Input: part model. Units: mm. Frame: model coordinates. A direction names the side the tool comes from. Coordinates: 2 decimals unless noted, no trailing zeros. Order: outer loops, then holes, each group sorted by start corner. A loop starts at its lowest first (then second) coordinate and runs counter-clockwise, first axis right, second up. Notation, with made-up numbers: (75, 54.5) - (112, 54.5) arc R8 cw to (112, 67.5) - close; hole circle Ø10 at (-7.5, -18). An arc over 180 degrees is marked (long way). Answer as CSV lines item,"result". Start each with the question number.
Item 1: Section A-A (z = -38). Output: boundary loops of the cut face in (x, y).
Item 2: Access query for faces 4 (the flat face through (44.8, -33.6, -1.4)), 5 (the flat face through (46, 8, -13)), 6 (the flat face through (0, 0, -5)). Directions: +Z, -Z, +X, -X, +Y, -Y. A direction counts if a zero-diameter tool reaches every point of the face in a straight line with its end or side. Return the directions, or none.
Item 3: First-contact query: pin 1 (4 mm diameter, centred on y = 12.5, z = -13.5, fed in from +X); pin 2 (5 mm diameter, centred on x = -11, z = -41.5, fed in from +Y); pin 3 (5 mm diameter, centred on y = -22.5, z = -21, fed in from +X). Flat tips, straight axial feed; report the tip coordinate or a pass-through.
Item 4: Material intervals for line 1 along Y through (x, z) = (0, -3.3); line 2 along Y through (x, z) = (0, -1.7); line 3 along X through (y, z) = (0, -46), sorted ascending.
Item 5: Draft query along Y for faces 1 (the flat face through (22, 34, -69)), 2 (the cylindrical face through (20.633, -15.821, -2.479)), 3 (the flat face through (22, -35, -35)). Return one class per face: +Y half, -Y half, draft (parallel to the pull), parting line (faces both ways), or undercut.
Item 6: Section B-B (y = 0). Output: boundary loops of the cut face in (x, z), and give its area (3 significant figures).
from build123d import *

# Parameters (mm, degrees)
BOSS_EXTRUDE1_DEPTH = 70
SKETCH4_R           = 25
BOSS_EXTRUDE2_DEPTH = 5
CHAMFER1_SIZE       = 2
SKETCH5_R           = 26
CUT_EXTRUDE1_DEPTH  = 5
CHAMFER3_SIZE       = 1


with BuildPart() as part:
    # Sketch3 → Boss-Extrude1 (new body)
    with BuildSketch(Plane.XY):
        with BuildLine():
            Line((0, 35), (46, 35))
            Line((46, 35), (46, -35))
            Line((46, -35), (0, -35))
            ThreePointArc((0, -35), (-35, 0), (0, 35))
        make_face()
    extrude(amount=BOSS_EXTRUDE1_DEPTH)

    # Sketch4 → Boss-Extrude2 (add)
    with BuildSketch(Plane(origin=(46, 0, 0), x_dir=(0, 0, -1), z_dir=(1, 0, 0))):
        with Locations(Location((-38, 0, 0), (0, 0, 180))):
            Circle(SKETCH4_R)
    extrude(amount=BOSS_EXTRUDE2_DEPTH)

    # Chamfer1
    chamfer1_edges = [part.edges().sort_by_distance(p)[0] for p in [
        (46, 0, 70),
        (23, 35, 70),
        (-35, 0, 70),
        (23, 35, 0),
        (46, 0, 0),
        (23, -35, 0),
        (-35, 0, 0),
        (23, -35, 70),
        (46, 35, 35),
        (46, -35, 35),
    ]]
    chamfer(chamfer1_edges, length=CHAMFER1_SIZE)

    # Sketch5 → Cut-Extrude1 (cut)
    with BuildSketch(Plane(origin=(0, 0, 0), x_dir=(-1, 0, 0), z_dir=(0, 0, -1))):
        Circle(SKETCH5_R)
    extrude(amount=-CUT_EXTRUDE1_DEPTH, mode=Mode.SUBTRACT)

    # Chamfer3
    chamfer3_edges = [part.edges().sort_by_distance(p)[0] for p in [
        (46, 0, 13),
        (51, 0, 13),
        (26, 0, 5),
        (26, 0, 0),
    ]]
    chamfer(chamfer3_edges, length=CHAMFER3_SIZE)


with BuildPart() as body_2:
    # Mirror1: mirrored copy
    add(part.part.mirror(Plane.XY))


solid = body_2.part
Determined:
1,outline,"(0, -35) - (44, -35) - (46, -33) - (46, -26) - (47, -25) - (50, -25) - (51, -24) - (51, 24) - (50, 25) - (47, 25) - (46, 26) - (46, 33) - (44, 35) - (0, 35) arc R35 ccw to start"
2,face 4,"+Z, +X, -Y"
2,face 5,"+X"
2,face 6,"+Z"
3,pin 1,"stops at x = 46.5"
3,pin 2,"stops at y = 33.95"
3,pin 3,"stops at x = 46.3"
4,line 1,"y = -35 to -26, 26 to 35"
4,line 2,"y = -34.7 to -26, 26 to 34.7"
4,line 3,"x = -35 to 51"
5,face 1,"+Y half"
5,face 2,"undercut"
5,face 3,"-Y half"
6,outline,"(-35, -68) - (-33, -70) - (44, -70) - (46, -68) - (46, -64) - (47, -63) - (50, -63) - (51, -62) - (51, -14) - (50, -13) - (47, -13) - (46, -12) - (46, -2) - (44, 0) - (27, 0) - (26, -1) - (26, -4) - (25, -5) - (-25, -5) - (-26, -4) - (-26, -1) - (-27, 0) - (-33, 0) - (-35, -2) - close"
6,area,"5,650 mm^2"
